```python
from build123d import *

# Parameters (mm, degrees)
EXTRUDE015_DEPTH = 1
EXTRUDE014_DEPTH = 2.25


with BuildPart() as extrude015:
    # Sketch015 → Extrude015 (new body)
    with BuildSketch(Plane.XZ):
        with BuildLine():
            ThreePointArc((11.7, 16.35), (11.063604, 16.086396), (10.8, 15.45))
            Line((10.8, 14.2), (10.8, 15.45))
            ThreePointArc((10.8, 14.2), (11.23934, 13.13934), (12.3, 12.7))
            Line((16.8, 12.7), (12.3, 12.7))
            ThreePointArc((16.8, 12.7), (17.86066, 13.13934), (18.3, 14.2))
            Line((18.3, 15.45), (18.3, 14.2))
            ThreePointArc((18.3, 15.45), (18.036396, 16.086396), (17.4, 16.35))
            Line((11.7, 16.35), (17.4, 16.35))
        make_face()
    extrude(amount=EXTRUDE015_DEPTH)


with BuildPart() as extrude015_1:
    # Extrude015 placement: moved
    add(extrude015.part.moved(Location((0, 3, 0))))


with BuildPart() as button1:
    # Sketch014 → Extrude014 (new body)
    with BuildSketch(Plane.XZ):
        with BuildLine():
            ThreePointArc((12.4, 16.25), (11.763604, 15.986396), (11.5, 15.35))
            Line((11.5, 14.3), (11.5, 15.35))
            ThreePointArc((11.5, 14.3), (11.763604, 13.663604), (12.4, 13.4))
            Line((16.7, 13.4), (12.4, 13.4))
            ThreePointArc((16.7, 13.4), (17.336396, 13.663604), (17.6, 14.3))
            Line((17.6, 15.35), (17.6, 14.3))
            ThreePointArc((17.6, 15.35), (17.336396, 15.986396), (16.7, 16.25))
            Line((12.4, 16.25), (16.7, 16.25))
        make_face()
    extrude(amount=EXTRUDE014_DEPTH)


with BuildPart() as button1_1:
    # Extrude014 placement: moved
    add(button1.part.moved(Location((0, 2, 0))))

    # Fusion018: union Extrude015
    add(extrude015_1.part)


solid = button1_1.part
```
Geometry check sheet. Reference: the model listing, model coordinates, mm. A direction names the side the tool comes from. Give positions to 0.01 mm unless a question says otherwise; leave off trailing zeros. Order: outer loops, then holes, each group sorted by start corner. A loop starts at its lowest first (then second) coordinate and runs counter-clockwise, first axis right, second up.
1. Section check C-C, the plane z = 13.3. Enter the section's corners in (x, y).
2. Thickness scan on L1, parallel to Y at x = 13, z = 13.05; L2, parallel to Z at x = 15.5, y = 0; L3, parallel to Z at x = 17.25, y = 2.1. Record the ranges inside material, lowest first.
3. Section check B-B, the plane x = 17.25. Enter the section's corners in (y, z).
4. Gauge pin test, flat ends, axial feed: pin 1 Ø0.7 at (x, y) = (14.5, 1.5) entering from +Z; pin 2 Ø0.7 at (x, y) = (14.5, 1) entering from -Z; pin 3 Ø1.2 at (y, z) = (1, 15) entering from +X. Record the tip position at first contact, or that the pin passes through.
5. Section check A-A, the plane y = 2.45. Enter the section's corners in (x, z).
6. Access from +Z, -Z, +X, -X, +Y, -Y to the whole of each face (thin tool, end or side, straight path). Record for faces 1 (the face through (17.6, 1, 15)), 2 (the face through (11.76, 0.89, 13.67)), 3 (the face through (15, 1, 16.25)).
Values follow:
1. outline: (11.1, 2) - (18, 2) - (18, 3) - (11.1, 3) - close
2. L1: y = 2 to 3
2. L2: z = 13.4 to 16.25
2. L3: z = 12.77 to 16.35
3. outline: (-0.25, 13.59) - (2, 13.59) - (2, 12.77) - (3, 12.77) - (3, 16.35) - (2, 16.35) - (2, 16.06) - (-0.25, 16.06) - close
4. pin 1: stops at z = 16.25
4. pin 2: stops at z = 13.4
4. pin 3: stops at x = 17.6
5. outline: (10.8, 14.2) arc R1.5 ccw to (12.3, 12.7) - (16.8, 12.7) arc R1.5 ccw to (18.3, 14.2) - (18.3, 15.45) arc R0.9 ccw to (17.4, 16.35) - (11.7, 16.35) arc R0.9 ccw to (10.8, 15.45) - close
6. face 1: +Z, -Z, +X, -Y
6. face 2: -Z, -X, -Y
6. face 3: +Z, +X, -X, -Y
